from build123d import *

# Parameters (mm, degrees)
SKETCH1_R           = 26
SKETCH1_R_2         = 23.625
BOSS_EXTRUDE1_DEPTH = 6
SKETCH2_W           = 7.25
SKETCH2_H           = 6
BOSS_EXTRUDE2_DEPTH = 6
CIRPATTERN1_COUNT   = 4
SKETCH3_R           = 2.5
CUT_EXTRUDE1_DEPTH  = 1.5
CIRPATTERN2_COUNT   = 4
FILLET1_R           = 1
SKETCH4_R           = 1.5
CUT_EXTRUDE2_DEPTH  = 4
CIRPATTERN4_COUNT   = 4


with BuildPart() as part:
    # Sketch1 → Boss-Extrude1 (new body)
    with BuildSketch(Plane(origin=(0, 0, 0), x_dir=(1, 0, 0), z_dir=(0, 1, 0))):
        Circle(SKETCH1_R)
        Circle(SKETCH1_R_2, mode=Mode.SUBTRACT)
    extrude(amount=BOSS_EXTRUDE1_DEPTH)

    # Sketch2 → Boss-Extrude2 (add)
    with BuildSketch(Plane(origin=(0, 6, 0), x_dir=(1, 0, 0), z_dir=(0, 1, 0))):
        with Locations((-22.20134314, 0)):
            Rectangle(SKETCH2_W, SKETCH2_H)
    boss_extrude2 = extrude(amount=-BOSS_EXTRUDE2_DEPTH)

    # CirPattern1: Boss-Extrude2 ×4 about axis
    cirpattern1_axis = Axis((0, 0, 0), (0, 1, 0))
    for i in range(1, CIRPATTERN1_COUNT):
        add(boss_extrude2.rotate(cirpattern1_axis, i * 360 / CIRPATTERN1_COUNT))

    # Sketch3 → Cut-Extrude1 (cut)
    with BuildSketch(Plane(origin=(-18.57634314, 0, 0), x_dir=(0, 0, -1), z_dir=(1, 0, 0))):
        with Locations((0, 6)):
            Circle(SKETCH3_R)
        Circle(SKETCH3_R)
    cut_extrude1 = extrude(amount=-CUT_EXTRUDE1_DEPTH, mode=Mode.SUBTRACT)

    # CirPattern2: Cut-Extrude1 ×4 about axis
    cirpattern2_axis = Axis((0, 0, 0), (0, 1, 0))
    for i in range(1, CIRPATTERN2_COUNT):
        add(cut_extrude1.rotate(cirpattern2_axis, i * 360 / CIRPATTERN2_COUNT), mode=Mode.SUBTRACT)

    # Fillet1
    fillet1_edges = [part.edges().sort_by_distance(p)[0] for p in [
        (-21.00504642, 6, 3),
        (-21.00504642, 6, -3),
        (-21.00504642, 0, -3),
        (-21.00504642, 0, 3),
        (3, 6, 21.00504642),
        (-3, 6, 21.00504642),
        (-3, 0, 21.00504642),
        (3, 0, 21.00504642),
        (21.00504642, 6, -3),
        (21.00504642, 6, 3),
        (21.00504642, 0, 3),
        (21.00504642, 0, -3),
        (-3, 6, -21.00504642),
        (3, 6, -21.00504642),
        (3, 0, -21.00504642),
        (-3, 0, -21.00504642),
    ]]
    fillet(fillet1_edges, radius=FILLET1_R)

    # Sketch4 → Cut-Extrude2 (cut)
    with BuildSketch(Plane.XY.offset(26)):
        with Locations((0, 3)):
            Circle(SKETCH4_R)
    cut_extrude2 = extrude(amount=-CUT_EXTRUDE2_DEPTH, mode=Mode.SUBTRACT)

    # CirPattern4: Cut-Extrude2 ×4 about axis
    cirpattern4_axis = Axis((0, 0, 0), (0, 1, 0))
    for i in range(1, CIRPATTERN4_COUNT):
        add(cut_extrude2.rotate(cirpattern4_axis, i * 360 / CIRPATTERN4_COUNT), mode=Mode.SUBTRACT)


solid = part.part
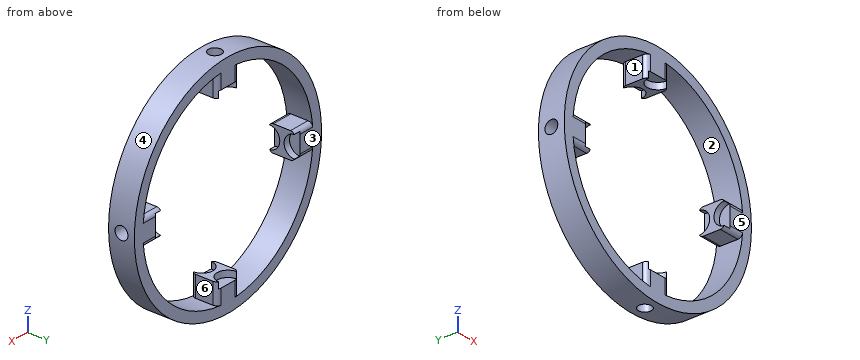
Read the model definition and answer for the solid it produces. Units are mm, in the model's axes. Face numbers are marked on the shaded views. A direction names the side the tool comes from. Round coordinates to 2 decimals unless told otherwise and drop trailing zeros. Order: outer loops, then holes, each group sorted by start corner. A loop starts at its lowest first (then second) coordinate and runs counter-clockwise, first axis right, second up.
1) Straight lines are drawn through the part: L1, parallel to X at y = 5.5, z = -20.5; L2, parallel to Y at x = 23, z = 0; L3, parallel to Z at x = 20, y = 4.25. For each, find the intervals that lie inside material, in ascending order.
2) The mould has two halves that part along X. Classify the marked faces 1, 2, 3 and 4: released by +X, released by -X, zero draft, split by the parting line, or undercut.
3) The part is cut by section D-D on z = -9.5. Write down the section's boundary in (x, y).
4) The part is cut by section B-B on z = 0. Write down the section's boundary in (x, y), plus the area to 3 significant figures.
5) For the marked faces 5 and 6, determine the directions among +Z, -Z, +X, -X, +Y, -Y from which every point of the face is accessible in a straight line to the end or side of a thin tool.
6) Flat-ended cylindrical pins translate along their axes: pin 1 (2.5 mm diameter, centred on x = 0, y = 3, fed in from -Z); pin 2 (2.5 mm diameter, centred on y = 3, z = 0, fed in from +X); pin 3 (3 mm diameter, centred on x = -4.5, y = 4.5, fed in from +Z). Find the tip coordinate at first contact, or state that the pin passes through.
7) The part is cut by section C-C on x = -16.5. Write down the section's boundary in (y, z).
8) The part is cut by section A-A on x = 0. Write down the section's boundary in (y, z), plus the area to 3 significant figures.
Resolved:
1. L1: x = -15.99 to -11.74, -2.87 to 2.87, 11.74 to 15.99
1. L2: y = 0 to 1.5, 4.5 to 6
1. L3: z = -16.61 to -12.58, -3 to -1.79, 1.79 to 3, 12.58 to 16.61
2. face 1: undercut
2. face 2: undercut
2. face 3: zero draft
2. face 4: split by the parting line
3. outline: (-24.2, 0) - (-21.63, 0) - (-21.63, 6) - (-24.2, 6) - close; (21.63, 0) - (24.2, 0) - (24.2, 6) - (21.63, 6) - close
4. outline: (-26, 0) - (-20.08, 0) - (-20.08, 2.5) - (-18.58, 2.5) - (-18.58, 3.5) - (-20.08, 3.5) - (-20.08, 6) - (-26, 6) - (-26, 4.5) - (-22, 4.5) - (-22, 1.5) - (-26, 1.5) - close; (18.58, 2.5) - (20.08, 2.5) - (20.08, 0) - (26, 0) - (26, 1.5) - (22, 1.5) - (22, 4.5) - (26, 4.5) - (26, 6) - (20.08, 6) - (20.08, 3.5) - (18.58, 3.5) - close
4. area: 50.1 mm2
5. face 5: +Z, -Z, +X, -X, -Y
5. face 6: +Y, -Y
6. pin 1: stops at z = -22
6. pin 2: stops at x = 22
6. pin 3: stops at z = 25.83
7. outline: (0, -20.09) - (6, -20.09) - (6, -16.91) - (0, -16.91) - close; (0, 16.91) - (6, 16.91) - (6, 20.09) - (0, 20.09) - close
8. outline: (0, -26) - (1.5, -26) - (1.5, -22) - (4.5, -22) - (4.5, -26) - (6, -26) - (6, -20.08) - (3.5, -20.08) - (3.5, -18.58) - (2.5, -18.58) - (2.5, -20.08) - (0, -20.08) - close; (0, 20.08) - (2.5, 20.08) - (2.5, 18.58) - (3.5, 18.58) - (3.5, 20.08) - (6, 20.08) - (6, 26) - (4.5, 26) - (4.5, 22) - (1.5, 22) - (1.5, 26) - (0, 26) - close
8. area: 50.1 mm2
